```python
from build123d import *

# Parameters (mm, degrees)
F1_DEPTH = 25
F2_R     = 5
F3_DEPTH = 150


with BuildPart() as f1:
    # F0 (on Top) → F1 (new body)
    with BuildSketch(Plane.XY):
        Polygon((31.593338, 4.139638), (-99.612067, 4.139638), (-99.612067, -25.860362), (31.593338, -25.860362), (81.593338, -25.860362), (100.387933, -25.860362), (100.387933, -20.079653), (117.500933, -20.079653), (117.500933, -1.641072), (100.387933, -1.641072), (100.387933, 4.139638), (81.593338, 4.139638), align=None)
    extrude(amount=-F1_DEPTH)

    # F2 (on face) → F3 (cut)
    with BuildSketch(Plane(origin=(-99.612067, 0, 0), x_dir=(0, -1, 0), z_dir=(-1, 0, 0))):
        with Locations((10.860362, -8.104307)):
            Circle(F2_R)
    extrude(amount=-F3_DEPTH, mode=Mode.SUBTRACT)


solid = f1.part
```
Verification items for the finished model (mm, model axes). A direction names the side the tool comes from. Give positions to 0.01 mm unless a question says otherwise; leave off trailing zeros. Loops run counter-clockwise (first coordinate to the right, second up) from the corner with the lowest first, then second, coordinate; pieces in that order, holes last. Notation, with made-up numbers: M -7,78.5 L 17,78.5 A16 ccw 17,90.5 Z; hole C -20,16.5 d11. An arc over 180 degrees is marked long. One line per question, with ' | ' between items.
Item 1: Section check A-A, the plane z = -20. Record the cut outline in (x, y).
Completed:
outline: M -99.61,-25.86 L 100.39,-25.86 L 100.39,-20.08 L 117.5,-20.08 L 117.5,-1.64 L 100.39,-1.64 L 100.39,4.14 L -99.61,4.14 Z
Item 2: Section check D-D, the plane z = -10.25. Record the cut outline in (x, y).
Completed:
outline: M -99.61,-25.86 L 100.39,-25.86 L 100.39,-20.08 L 117.5,-20.08 L 117.5,-1.64 L 100.39,-1.64 L 100.39,4.14 L -99.61,4.14 L -99.61,-6.34 L 50.39,-6.34 L 50.39,-15.38 L -99.61,-15.38 Z
Item 3: Thickness scan on line 1 (X direction, y = 0.25, z = -6); line 2 (Z direction, x = -2.5, y = -6.5); line 3 (Y direction, x = -81, z = -5.25). Record the ranges inside material, lowest first. Write a range as [from, to].
Completed:
line 1: x = [-99.61, 100.39] | line 2: z = [-25, -10.55], [-5.66, 0] | line 3: y = [-25.86, -14.97], [-6.76, 4.14]
Item 4: Depth check by flat-ended pin: P1, Ø1.7, axis at y = 2.5, z = -7.5, coming from the +X side; P2, Ø4, axis at y = -8.5, z = -9.5, coming from the -X side. Enter the tip coordinate at first touch or a pass-through.
Completed:
P1: stops at x = 100.39 | P2: stops at x = 50.39
Item 5: Section check C-C, the plane y = -10.5. Record the cut outline in (x, z), plus the area to 3 significant figures.
Completed:
outline: M -99.61,-25 L 117.5,-25 L 117.5,0 L -99.61,0 L -99.61,-3.12 L 50.39,-3.12 L 50.39,-13.09 L -99.61,-13.09 Z | area: 3,930 mm^2
Item 6: Draft check along Y on faces 4 (the face through (-25.66, -15.48, -10.02)), 5 (the face through (100.388, 1, -12)), 6 (the face through (2, 4.14, -12)). Enter one of: +Y half, -Y half, draft (parallel to the pull), parting line (faces both ways), or undercut.
Completed:
face 4: undercut | face 5: draft | face 6: +Y half
Item 7: Section check B-B, the plane x = -55. Record the cut outline in (y, z).
Completed:
outline: M -25.86,-25 L 4.14,-25 L 4.14,0 L -25.86,0 Z; hole C -10.86,-8.1 d10
Item 8: Tool access check on faces 1 (the face through (109, -1.641, -12)), 2 (the face through (100.388, -23, -12)), 3 (the face through (50.388, -11, -8)). Record the directions out of +Z, -Z, +X, -X, +Y, -Y that give a thin tool (end or side, any length) a straight path to the whole face; none if there is none.
Completed:
face 1: +Z, -Z, +X, +Y | face 2: +Z, -Z, +X, -Y | face 3: -X
